from build123d import *
from OCP.BRepFilletAPI import BRepFilletAPI_MakeChamfer

# Parameters (mm, degrees)
AUFSATZ_LINEAR_AUSTRAGEN1_DEPTH                      = 6
SKIZZE8_W                                            = 32
SKIZZE8_H                                            = 50
AUFSATZ_LINEAR_AUSTRAGEN2_DEPTH                      = 4
SCHNITT_LINEAR_AUSTRAGEN1_DEPTH                      = 62.846584384
STIRNSENKUNG_F_R_M5_FLACHKOPFSCHRAUBE_MI_D           = 5.5
STIRNSENKUNG_F_R_M5_FLACHKOPFSCHRAUBE_MI_DEPTH       = 20
STIRNSENKUNG_F_R_M5_FLACHKOPFSCHRAUBE_MI_CBORE_D     = 11
STIRNSENKUNG_F_R_M5_FLACHKOPFSCHRAUBE_MI_CBORE_DEPTH = 1.7
STIRNSENKUNG_F_R_M5_FLACHKOPFSCHRAUBE_MI_TIP         = 1.652366702
FORMSENKUNG_F_R_M3_LINSENSENKSCHRAUBE_MI_D           = 3.4
FORMSENKUNG_F_R_M3_LINSENSENKSCHRAUBE_MI_DEPTH       = 8.5
FORMSENKUNG_F_R_M3_LINSENSENKSCHRAUBE_MI_CSINK_D     = 6.3
FORMSENKUNG_F_R_M3_LINSENSENKSCHRAUBE_MI_CSINK_ANGLE = 90
FORMSENKUNG_F_R_M3_LINSENSENKSCHRAUBE_MI_TIP         = 1.021463052
FASE1_SIZE                                           = 2
FASE1_SIZE2                                          = 2.233305694
VERRUNDUNG1_R                                        = 5
M4_GEWINDEBOHRUNG1_D                                 = 3.3
M4_GEWINDEBOHRUNG2_REACH                             = 80.333
M4_GEWINDEBOHRUNG2_BORE_R                            = 1.65


with BuildPart() as part:
    # Skizze1 → Aufsatz-Linear austragen1 (new body)
    with BuildSketch(Plane(origin=(0, 0, 0), x_dir=(1, 0, 0), z_dir=(0, 1, 0))):
        Polygon((-50, 35), (-29, 35), (-29, 25), (40, 25), (40, -25), (0, -25), (-50, -20), align=None)
    extrude(amount=AUFSATZ_LINEAR_AUSTRAGEN1_DEPTH)

    # Skizze8 → Aufsatz-Linear austragen2 (add)
    with BuildSketch(Plane.XZ):
        with Locations((24, 0)):
            Rectangle(SKIZZE8_W, SKIZZE8_H)
    extrude(amount=AUFSATZ_LINEAR_AUSTRAGEN2_DEPTH)

    # Skizze4 → Schnitt-Linear austragen1 (cut, through all)
    with BuildSketch(Plane(origin=(0, 6, 0), x_dir=(1, 0, 0), z_dir=(0, 1, 0))):
        with BuildLine():
            Line((11, 10.5), (11, -10.5))
            ThreePointArc((11, -10.5), (22, -21.5), (33, -10.5))
            Line((33, -10.5), (33, 10.5))
            ThreePointArc((33, 10.5), (22, 21.5), (11, 10.5))
        make_face()
    extrude(amount=-SCHNITT_LINEAR_AUSTRAGEN1_DEPTH, mode=Mode.SUBTRACT)

    # Stirnsenkung für M5 Flachkopfschraube mit Schlitz2
    with Locations(Plane(origin=(0, 0, 0), x_dir=(-1, 0, 0), z_dir=(0, -1, 0))):
        with Locations((35, 0)):
            CounterBoreHole(STIRNSENKUNG_F_R_M5_FLACHKOPFSCHRAUBE_MI_D / 2, STIRNSENKUNG_F_R_M5_FLACHKOPFSCHRAUBE_MI_CBORE_D / 2, STIRNSENKUNG_F_R_M5_FLACHKOPFSCHRAUBE_MI_CBORE_DEPTH, depth=STIRNSENKUNG_F_R_M5_FLACHKOPFSCHRAUBE_MI_DEPTH)
            with Locations((0, 0, -(STIRNSENKUNG_F_R_M5_FLACHKOPFSCHRAUBE_MI_DEPTH + STIRNSENKUNG_F_R_M5_FLACHKOPFSCHRAUBE_MI_TIP / 2))):  # 118° drill point
                Cone(0, STIRNSENKUNG_F_R_M5_FLACHKOPFSCHRAUBE_MI_D / 2, STIRNSENKUNG_F_R_M5_FLACHKOPFSCHRAUBE_MI_TIP, mode=Mode.SUBTRACT)

    # Formsenkung für M3 Linsensenkschraube mit Schlitz1
    with Locations(Plane(origin=(0, 6, 0), x_dir=(1, 0, 0), z_dir=(0, 1, 0))):
        with Locations((5.5, 8), (5.5, -8)):
            CounterSinkHole(FORMSENKUNG_F_R_M3_LINSENSENKSCHRAUBE_MI_D / 2, FORMSENKUNG_F_R_M3_LINSENSENKSCHRAUBE_MI_CSINK_D / 2, depth=FORMSENKUNG_F_R_M3_LINSENSENKSCHRAUBE_MI_DEPTH, counter_sink_angle=FORMSENKUNG_F_R_M3_LINSENSENKSCHRAUBE_MI_CSINK_ANGLE)
            with Locations((0, 0, -(FORMSENKUNG_F_R_M3_LINSENSENKSCHRAUBE_MI_DEPTH + FORMSENKUNG_F_R_M3_LINSENSENKSCHRAUBE_MI_TIP / 2))):  # 118° drill point
                Cone(0, FORMSENKUNG_F_R_M3_LINSENSENKSCHRAUBE_MI_D / 2, FORMSENKUNG_F_R_M3_LINSENSENKSCHRAUBE_MI_TIP, mode=Mode.SUBTRACT)

    # Fase1: one chamfer whose edges measure the first distance from different faces: ONE call of the kernel's chamfer builder (chamfer() names one face for all edges)
    fase1_edges_1 = [part.edges().sort_by_distance(p)[0] for p in [
        (40, 1, 25),
        (-50, 3, -35),
        (-29, 3, -35),
        (40, 1, -25),
    ]]
    fase1_edges_2 = [part.edges().sort_by_distance(p)[0] for p in [
        (-50, 3, 20),
    ]]
    fase1_side_2 = [part.faces().sort_by_distance(p)[0] for p in [
        (-50, 3, -7.5),
    ]]
    fase1 = BRepFilletAPI_MakeChamfer(part.part.solid().wrapped)
    for e in fase1_edges_1:
        fase1.Add(FASE1_SIZE, e.wrapped)
    for e in fase1_edges_2:
        fase1.Add(FASE1_SIZE, FASE1_SIZE2, e.wrapped, fase1_side_2[0].wrapped)  # the first distance lies on this face
    add(Compound.cast(fase1.Shape()), mode=Mode.REPLACE)

    # Verrundung1
    verrundung1_edges = [part.edges().sort_by_distance(p)[0] for p in [
        (-29, 3, -25),
    ]]
    fillet(verrundung1_edges, radius=VERRUNDUNG1_R)

    # M4 Gewindebohrung1 (through all)
    with Locations(Plane(origin=(0, 6, 0), x_dir=(1, 0, 0), z_dir=(0, 1, 0))):
        with Locations((-39.5, 25)):
            Hole(M4_GEWINDEBOHRUNG1_D / 2)

    # M4 Gewindebohrung2 bore → M4 Gewindebohrung2 (cut, up to next)
    with BuildSketch(Plane.XY.offset(25), mode=Mode.PRIVATE) as m4_gewindebohrung2_sk1:
        with Locations((22, 1)):
            Circle(M4_GEWINDEBOHRUNG2_BORE_R)
    m4_gewindebohrung2_tool1 = extrude(m4_gewindebohrung2_sk1.sketch, amount=-M4_GEWINDEBOHRUNG2_REACH, mode=Mode.PRIVATE) & part.part
    add(m4_gewindebohrung2_tool1.solids().sort_by_distance((22, 1, 25))[0], mode=Mode.SUBTRACT)


solid = part.part
Read the model definition and answer for the solid it produces. Units are mm, in the model's axes. A direction names the side the tool comes from. Round coordinates to 2 decimals unless told otherwise and drop trailing zeros. Order: outer loops, then holes, each group sorted by start corner. A loop starts at its lowest first (then second) coordinate and runs counter-clockwise, first axis right, second up.
1) The mould has two halves that part along Z. Classify faces 1 (the face through (-36, 1.7, -3)), 2 (the face through (39, 1, 24)), 3 (the face through (20.35, 1.07, 23.21)), 4 (the face through (13, 2, -25)): released by +Z, released by -Z, zero draft, split by the parting line, or undercut.
2) The part is cut by section A-A on z = 0. Write down the section's boundary in (x, y).
3) The part is cut by section B-B on x = 5.5. Write down the section's boundary in (y, z), plus the area to 3 significant figures.
4) The part is cut by section D-D on z = -13.5. Write down the section's boundary in (x, y), plus the area to 3 significant figures.
5) Flat-ended cylindrical pins translate along their axes: pin 1 (4.5 mm diameter, centred on x = -39.5, z = -25, fed in from -Y); pin 2 (2.5 mm diameter, centred on y = 2, z = -31, fed in from +X); pin 3 (1.2 mm diameter, centred on y = -1, z = -1.5, fed in from -X); pin 4 (3 mm diameter, centred on x = 5.5, z = -8, fed in from +Y). Find the tip coordinate at first contact, or state that the pin passes through.
6) Straight lines are drawn through the part: L1, parallel to Z at x = 5.5, y = 3.05; L2, parallel to X at y = -1.25, z = 8.5; L3, parallel to X at y = 2.5, z = 8. For each, find the intervals that lie inside material, in ascending order.
7) The part is cut by section C-C on y = -2.25. Write down the section's boundary in (x, z).
8) For faces 5 (the face through (-29.505, 0.838, -0.242)), 6 (the face through (22.2, 1.1, -21.5)), 7 (the face through (-21, 0, -5)), determine the directions among +Z, -Z, +X, -X, +Y, -Y from which every point of the face is accessible in a straight line to the end or side of a thin tool.
Resolved:
1. face 1: undercut
1. face 2: released by +Z
1. face 3: zero draft
1. face 4: released by -Z
2. outline: (-50, 0) - (-40.5, 0) - (-40.5, 1.7) - (-37.75, 1.7) - (-37.75, 6) - (-50, 6) - close; (-32.25, 1.7) - (-29.5, 1.7) - (-29.5, 0) - (8, 0) - (8, -4) - (11, -4) - (11, 6) - (-32.25, 6) - close; (33, -4) - (40, -4) - (40, 6) - (33, 6) - close
3. outline: (0, -25) - (6, -25) - (6, -11.15) - (4.55, -9.7) - (0, -9.7) - close; (0, -6.3) - (4.55, -6.3) - (6, -4.85) - (6, 4.85) - (4.55, 6.3) - (0, 6.3) - close; (0, 9.7) - (4.55, 9.7) - (6, 11.15) - (6, 25) - (0, 25) - close
3. area: 255 mm2
4. outline: (-50, 0) - (8, 0) - (8, -4) - (11.42, -4) - (11.42, 6) - (-50, 6) - close; (32.58, -4) - (40, -4) - (40, 6) - (32.58, 6) - close
4. area: 456 mm2
5. pin 1: stops at y = 0
5. pin 2: stops at x = -28.99
5. pin 3: stops at x = 8
5. pin 4: passes through
6. L1: z = -25 to -9.7, -6.3 to 6.3, 9.7 to 25
6. L2: x = 8 to 11, 33 to 40
6. L3: x = -50 to 3.8, 7.2 to 11, 33 to 40
7. outline: (8, -25) - (38, -25) - (40, -23) - (40, 23) - (38, 25) - (8, 25) - close; hole (11, -10.5) arc R11 ccw to (33, -10.5) - (33, 10.5) arc R11 ccw to (11, 10.5) - close
8. face 5: -Y
8. face 6: +Y, -Y
8. face 7: +Z, -Z, -X, -Y
